Geometry: see drawing. Coordinates: mm, zero at the bounding-box minimum. Coordinates: 2 decimals unless noted, no trailing zeros. Write each loop counter-clockwise with the first axis right and the second up, starting at its lowest first coordinate (ties: lowest second). Pieces come first, ordered by that corner, then holes. Notation, with made-up numbers: (51, 69.25) - (64, 69.25) arc R24 ccw to (64, 106.25) - close; hole circle Ø8 at (-8.75, -32). An arc over 180 degrees is marked (long way). One line per question, with ' | ' between items. Start each with the question number.
Q1. Line query: line 1 (X direction, y = 19.15, z = 1.85); line 2 (Y direction, x = 12, z = 2.45); line 3 (X direction, y = 18.5, z = 0.6). Output: solid intervals per line, ascending.
Q2. Cut plane C-C, the plane z = 1.4. Return loops of the section in (x, y).
Q3. Cut plane B-B, the plane y = 19.15. Return loops of the section in (x, z) (3 decimals), plus the area to 3 significant figures.
Q4. Draft query along X for the marked faces 1, 2, 3 and 4. Return one class per face: +X half, -X half, draft (parallel to the pull), parting line (faces both ways), or undercut.
Q5. Cut plane D-D, the plane y = 4. Return loops of the section in (x, z) (3 decimals), plus the area to 3 significant figures.
Q6. Cut plane A-A, the plane x = 4. Return loops of the section in (y, z) (3 decimals).
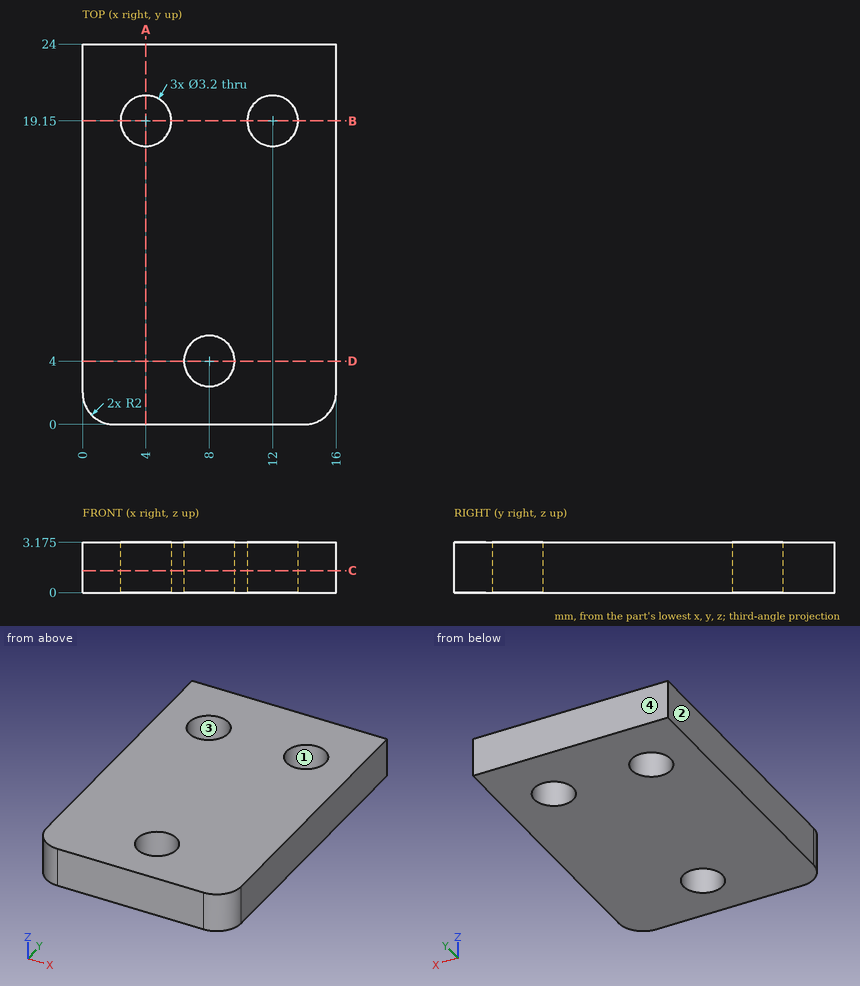
Reply:
1) line 1: x = 0 to 2.4, 5.6 to 10.4, 13.6 to 16 | line 2: y = 0 to 17.55, 20.75 to 24 | line 3: x = 0 to 2.54, 5.46 to 10.54, 13.46 to 16
2) outline: (0, 2) arc R2 ccw to (2, 0) - (14, 0) arc R2 ccw to (16, 2) - (16, 24) - (0, 24) - close; hole circle Ø3.2 at (4, 19.15); hole circle Ø3.2 at (8, 4); hole circle Ø3.2 at (12, 19.15)
3) outline: (0, 0) - (2.4, 0) - (2.4, 3.175) - (0, 3.175) - close; (5.6, 0) - (10.4, 0) - (10.4, 3.175) - (5.6, 3.175) - close; (13.6, 0) - (16, 0) - (16, 3.175) - (13.6, 3.175) - close | area: 30.5 mm^2
4) face 1: undercut | face 2: -X half | face 3: undercut | face 4: draft
5) outline: (0, 0) - (6.4, 0) - (6.4, 3.175) - (0, 3.175) - close; (9.6, 0) - (16, 0) - (16, 3.175) - (9.6, 3.175) - close | area: 40.6 mm^2
6) outline: (0, 0) - (17.55, 0) - (17.55, 3.175) - (0, 3.175) - close; (20.75, 0) - (24, 0) - (24, 3.175) - (20.75, 3.175) - close
